Input: part model. Units: mm. Frame: model coordinates. Face numbers are marked on the shaded views. A direction names the side the tool comes from. Coordinates: 2 decimals unless noted, no trailing zeros. Write each loop counter-clockwise with the first axis right and the second up, starting at its lowest first coordinate (ties: lowest second). Pieces come first, ordered by that corner, then holes. Notation, with made-up numbers: (72.5, 31.5) - (93.5, 31.5) arc R20 cw to (93.5, 66.5) - close; hole circle Ø1 at (-34, -1). An arc over 180 degrees is marked (long way). Put each result on its own line as item: value. Start each with the question number.
1. Cut plane B-B, the plane z = 75. Return loops of the section in (x, y), and give its area (3 significant figures).
2. Cut plane A-A, the plane y = 19. Return loops of the section in (x, z), and give its area (3 significant figures).
3. Line query: line 1 (X direction, y = 19.25, z = -83.5); line 2 (Y direction, x = 1, z = -45). Output: solid intervals per line, ascending.
4. Access query for the marked faces 1 and 2. Directions: +Z, -Z, +X, -X, +Y, -Y. A direction counts if a zero-diameter tool reaches every point of the face in a straight line with its end or side. Return the directions, or none.
5. Pin query (flat end, axial travel): pin 1 (6 mm diameter, centred on x = -2.5, z = -27.5, fed in from +Y). Return the tip coordinate at first contact, or that it passes through.
6. Cut plane C-C, the plane x = -4. Return loops of the section in (y, z).
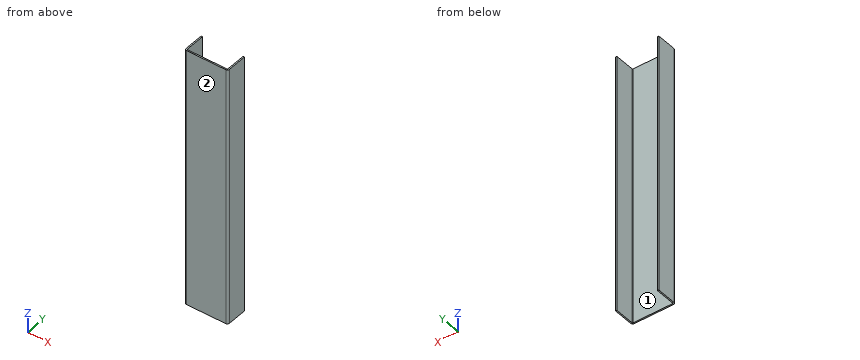
from build123d import *

# Parameters (mm, degrees)
SKETCH1_W                    = 50.8
SKETCH1_H                    = 304.8
BASE_FLANGE1_DEPTH           = 1.5875
EDGE_FLANGE1_STRIP_W         = 7.8232
EDGE_FLANGE1_STRIP_H         = 1.5875
EDGE_FLANGE1_STRIP_CUT_DEPTH = 304.8
EDGE_FLANGE1_DEPTH           = 304.8
EDGE_FLANGE2_STRIP_W         = 7.8232
EDGE_FLANGE2_STRIP_H         = 1.5875
EDGE_FLANGE2_STRIP_CUT_DEPTH = 304.8
EDGE_FLANGE2_DEPTH           = 304.8


# Sheet-metal steps are written as plain solids
with BuildPart() as part:
    # Sketch1 → Base-Flange1 (new body)
    with BuildSketch(Plane(origin=(0, 0, 0), x_dir=(1, 0, 0), z_dir=(0, 1, 0))):
        Rectangle(SKETCH1_W, SKETCH1_H)
    extrude(amount=-BASE_FLANGE1_DEPTH)

    # Edge-Flange1 strip (across the edge) → Edge-Flange1 strip cut (cut)
    with BuildSketch(Plane(origin=(25.4, 0, 152.4), x_dir=(-1, 0, 0), z_dir=(0, 0, -1))):
        with Locations((-1.5875, -0.79375)):
            Rectangle(EDGE_FLANGE1_STRIP_W, EDGE_FLANGE1_STRIP_H)
    extrude(amount=EDGE_FLANGE1_STRIP_CUT_DEPTH, mode=Mode.SUBTRACT)

    # Edge-Flange1 section (across the edge) → Edge-Flange1 (add)
    with BuildSketch(Plane(origin=(25.4, 0, 152.4), x_dir=(-1, 0, 0), z_dir=(0, 0, -1))):
        with BuildLine():
            Line((0, 0.7366), (0, 23.8125))
            Line((0, 23.8125), (1.5875, 23.8125))
            Line((1.5875, 23.8125), (1.5875, 0.7366))
            ThreePointArc((1.5875, 0.7366), (1.803245145, 0.215745145), (2.3241, 0))
            Line((2.3241, 0), (2.3241, -1.5875))
            ThreePointArc((2.3241, -1.5875), (0.68071313, -0.90678687), (0, 0.7366))
        make_face()
    extrude(amount=EDGE_FLANGE1_DEPTH)

    # Edge-Flange2 strip (across the edge) → Edge-Flange2 strip cut (cut)
    with BuildSketch(Plane(origin=(-25.4, 0, -152.4), x_dir=(1, 0, 0), z_dir=(0, 0, 1))):
        with Locations((-1.5875, -0.79375)):
            Rectangle(EDGE_FLANGE2_STRIP_W, EDGE_FLANGE2_STRIP_H)
    extrude(amount=EDGE_FLANGE2_STRIP_CUT_DEPTH, mode=Mode.SUBTRACT)

    # Edge-Flange2 section (across the edge) → Edge-Flange2 (add)
    with BuildSketch(Plane(origin=(-25.4, 0, -152.4), x_dir=(1, 0, 0), z_dir=(0, 0, 1))):
        with BuildLine():
            Line((0, 0.7366), (0, 23.8125))
            Line((0, 23.8125), (1.5875, 23.8125))
            Line((1.5875, 23.8125), (1.5875, 0.7366))
            ThreePointArc((1.5875, 0.7366), (1.803245145, 0.215745145), (2.3241, 0))
            Line((2.3241, 0), (2.3241, -1.5875))
            ThreePointArc((2.3241, -1.5875), (0.68071313, -0.90678687), (0, 0.7366))
        make_face()
    extrude(amount=EDGE_FLANGE2_DEPTH)


solid = part.part
Report:
1. outline: (-25.4, 0.74) arc R2.32 ccw to (-23.08, -1.59) - (23.08, -1.59) arc R2.32 ccw to (25.4, 0.74) - (25.4, 23.81) - (23.81, 23.81) - (23.81, 0.74) arc R0.74 cw to (23.08, 0) - (-23.08, 0) arc R0.74 cw to (-23.81, 0.74) - (-23.81, 23.81) - (-25.4, 23.81) - close
1. area: 154 mm^2
2. outline: (-25.4, -152.4) - (-23.81, -152.4) - (-23.81, 152.4) - (-25.4, 152.4) - close; (23.81, -152.4) - (25.4, -152.4) - (25.4, 152.4) - (23.81, 152.4) - close
2. area: 968 mm^2
3. line 1: x = -25.4 to -23.81, 23.81 to 25.4
3. line 2: y = -1.59 to 0
4. face 1: +Z, -Z, +Y
4. face 2: +Z, -Z, +X, -X, -Y
5. pin 1: stops at y = 0
6. outline: (-1.59, -152.4) - (0, -152.4) - (0, 152.4) - (-1.59, 152.4) - close
